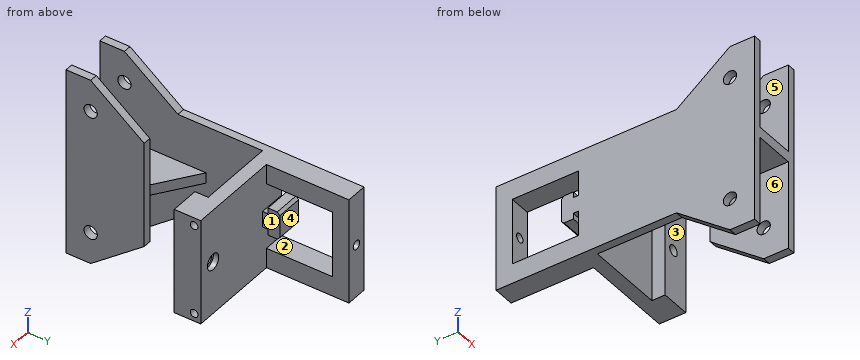
Autodesk Inventor part; units mm, degrees
ref_plane "YZ Plane" through (0, 0, 0) normal (1, 0, 0) x (0, 1, 0)
ref_plane "XZ Plane" through (0, 0, 0) normal (0, 1, 0) x (-1, 0, 0)
ref_plane "XY Plane" through (0, 0, 0) normal (0, 0, 1) x (1, 0, 0)
sketch "Szkic1" plane through (0, 0, 0) normal (1, 0, 0) x (0, 1, 0)
  line L0 (81.6216, 12.5) -> (106.6216, 12.5)
  line L1 (106.6216, 12.5) -> (106.6216, -12.5)
  line L2 (106.6216, -12.5) -> (81.6216, -12.5)
  line L3 (81.6216, -12.5) -> (81.6216, 12.5)
  line L4 (81.6216, 12.5) -> (106.6216, -12.5) construction
  line L5 (106.6216, 12.5) -> (81.6216, -12.5) construction
  line L6 (112.7335, 0) -> (112.7335, 20)
  line L7 (112.7335, 20) -> (44.7131, 20)
  line L8 (44.7131, 20) -> (24.5326, 35.4833)
  line L9 (24.5326, 35.4833) -> (15.2555, 35.4833)
  line L10 (15.2555, 35.4833) -> (15.2555, 0)
  line L11 (112.7335, 0) -> (112.7335, -20)
  line L12 (112.7335, -20) -> (44.7131, -20)
  line L13 (44.7131, -20) -> (24.5326, -35.4833)
  line L14 (24.5326, -35.4833) -> (15.2555, -35.4833)
  line L15 (15.2555, -35.4833) -> (15.2555, 0)
  point P0 (0, 0)
  point P1 (94.1216, 0)
  point P2 (24.5326, 19.6832)
  point P3 (24.5326, -19.6832)
  dimension "d0" = 25
  dimension "d1" = 25
  dimension "d2" = 82.089
  dimension "d3" = 20
extrude "Wyciągnięcie proste1" add sketch "Szkic1" along normal blind 3
sketch "Szkic2" plane through (3, 0, 0) normal (1, 0, 0) x (0, 0, -1)
  line L0 (-12.5, 106.6216) -> (12.5, 106.6216)
  line L1 (-35.4833, 24.5326) -> (-35.4833, 15.2555)
  line L2 (35.4833, 15.2555) -> (35.4833, 24.5326)
  point P0 (0, 0)
  point P1 (-23.4833, 24.5326)
  point P2 (23.4833, 24.5326)
  dimension "d6" = 82.089
  dimension "d7" = 82.089
  dimension "d8" = 12
  dimension "d9" = 12
hole "Otwór1" at (3, 24.5326, 23.4833) at (3, 24.5326, -23.4833) direction (-1, 0, 0) diameter 5 depth 3
sketch "Szkic3" plane through (3, 0, 0) normal (1, 0, 0) x (0, 0, -1)
  line L0 (-12.5, 106.6216) -> (12.5, 106.6216)
  line L1 (-12.5, 106.6216) -> (-20, 106.6216)
  line L2 (-20, 112.7335) -> (-20, 44.7131)
  line L3 (-12.5, 81.6216) -> (-12.5, 106.6216)
  line L4 (-20, 81.6216) -> (-12.5, 81.6216)
  line L5 (-12.5, 81.6216) -> (-12.5, 106.6216)
  line L6 (12.5, 106.6216) -> (12.5, 81.6216)
  line L7 (12.5, 106.6216) -> (12.5, 81.6216)
  line L8 (12.5, 81.6216) -> (20, 81.6216)
  line L9 (20, 81.6216) -> (20, 106.6216)
  line L10 (20, 106.6216) -> (12.5, 106.6216)
  line L11 (20, 44.7131) -> (20, 112.7335)
  point P0 (0, 0)
  point P1 (-20, 81.6216)
  dimension "d36" = 0
extrude "Wyciągnięcie proste2" add sketch "Szkic3" along normal blind 5
sketch "Szkic5" plane through (3, 0, 0) normal (1, 0, 0) x (0, 0, -1)
  line L0 (-35.4833, 15.2555) -> (35.4833, 15.2555)
  line L1 (0, 15.2555) -> (-2, 15.2555)
  line L2 (-2, 15.2555) -> (-2, 55.2555)
  line L3 (-2, 55.2555) -> (2, 55.2555)
  line L4 (2, 55.2555) -> (2, 15.2555)
  line L5 (0, 15.2555) -> (2, 15.2555)
  point P0 (0, 0)
  dimension "d26" = 2
  dimension "d27" = 40
  dimension "d28" = 4
extrude "Wyciągnięcie proste3" add sketch "Szkic5" along normal blind 15
sketch "Szkic6" plane through (18, 0, 0) normal (1, 0, 0) x (0, 0, -1)
  line L0 (-35.4833, 15.2555) -> (35.4833, 15.2555)
  line L1 (35.4833, 15.2555) -> (35.4833, 24.5326)
  line L2 (-35.4833, 15.2555) -> (35.4833, 15.2555)
  line L3 (35.4833, 15.2555) -> (35.4833, 24.5326)
  line L4 (35.4833, 24.5326) -> (20, 44.7131)
  line L5 (35.4833, 24.5326) -> (20, 44.7131)
  line L6 (-20, 44.7131) -> (-35.4833, 24.5326)
  line L7 (20, 44.7131) -> (-20, 44.7131)
  line L8 (-35.4833, 24.5326) -> (-35.4833, 15.2555)
  line L9 (-20, 44.7131) -> (-35.4833, 24.5326)
  line L10 (-35.4833, 24.5326) -> (-35.4833, 15.2555)
  circle A0 centre (-23.4833, 24.5326) radius 2.5
  circle A1 centre (23.4833, 24.5326) radius 2.5
  point P0 (0, 0)
extrude "Wyciągnięcie proste4" add sketch "Szkic6" along normal blind 3
chamfer "Faza1" distance 10.542 distance2 15 1 edges at (18, 55.2555, 0) measured on face at (18, 51.7413, 0.6667)
sketch "Szkic7" plane through (3, 0, 0) normal (1, 0, 0) x (0, 0, -1)
  line L0 (-20, 81.6216) -> (-12.5, 81.6216)
  line L1 (20, 44.7131) -> (20, 112.7335)
  line L2 (-20, 81.6216) -> (20, 81.6216)
  line L3 (20, 81.6216) -> (20, 76.6216)
  line L4 (20, 76.6216) -> (-20, 76.6216)
  line L5 (-20, 76.6216) -> (-20, 81.6216)
  point P0 (0, 0)
  dimension "d37" = 5
extrude "Wyciągnięcie proste5" add sketch "Szkic7" along normal blind 40
sketch "Szkic8" plane through (0, 81.6216, 12.5) normal (0, 1, 0) x (1, 0, 0)
  point P0 (0, 12.5)
  point P1 (36.4571, 12.5)
hole "Otwór3" at (36.4571, 81.6216, 0) direction (0, -1, 0) diameter 4 end through all
sketch "Szkic9" plane through (3, 0, 0) normal (1, 0, 0) x (0, 0, -1)
  line L0 (20, 112.7335) -> (-20, 112.7335)
  line L1 (20, 106.6216) -> (12.5, 106.6216)
  line L2 (-20, 112.7335) -> (20, 112.7335)
  line L3 (20, 112.7335) -> (20, 106.6216)
  line L4 (20, 106.6216) -> (-20, 106.6216)
  line L5 (-20, 106.6216) -> (-20, 112.7335)
  point P0 (0, 0)
extrude "Wyciągnięcie proste6" add sketch "Szkic9" along normal up to surface (5 mm away)
sketch "Szkic10" plane through (0, 0, 0) normal (-1, 0, 0) x (0, 0, 1)
  line L0 (-3.025, 81.6216) -> (-3.025, 83.6216)
  line L1 (-3.025, 83.6216) -> (-5.25, 83.6216)
  line L2 (-5.25, 83.6216) -> (-5.25, 87.1216)
  line L3 (0, 88.1216) -> (-4.25, 88.1216)
  line L4 (-4.25, 88.1216) -> (-5.25, 87.1216)
  line L5 (0, 88.1216) -> (4.25, 88.1216)
  line L6 (4.25, 88.1216) -> (5.25, 87.1216)
  line L7 (5.25, 83.6216) -> (5.25, 87.1216)
  line L8 (3.025, 83.6216) -> (5.25, 83.6216)
  line L9 (3.025, 81.6216) -> (3.025, 83.6216)
  line L10 (-12.5, 81.6216) -> (12.5, 81.6216)
  point P0 (0, 0)
  point P1 (0, 81.6216)
  point P2 (0, 81.6216)
  point P3 (-3.025, 82.6216)
  dimension "d49" = 2
  dimension "d50" = 2.225
  dimension "d51" = 3.5
  dimension "d52" = 4.25
  dimension "d53" = 0
  dimension "d54" = 3.025
extrude "Wyciągnięcie proste7" add sketch "Szkic10" against normal blind 10
sketch "Szkic11" plane through (0, 112.7335, 20) normal (0, 1, 0) x (1, 0, 0)
  point P0 (0, 20)
  point P1 (4, 20)
hole "Otwór4" at (4, 112.7335, 0) direction (0, -1, 0) diameter 3.4 depth 6.1119
sketch "Szkic13" plane through (3, 76.6216, -20) normal (0, -1, 0) x (1, 0, 0)
  line L0 (0, 0) -> (40, 0)
  line L1 (40, 40) -> (29, 40)
  line L2 (29, 40) -> (29, 0)
  line L3 (29, 0) -> (40, 0)
  line L4 (40, 0) -> (40, 40)
  point P0 (-3, 20)
  dimension "d65" = 11
extrude "Wyciągnięcie proste8" add sketch "Szkic13" along normal blind 5
sketch "Szkic14" plane through (0, 81.6216, 12.5) normal (0, 1, 0) x (1, 0, 0)
  circle A0 centre (36.4571, 12.5) radius 2
  circle A1 centre (36.4571, 12.5) radius 2
  point P0 (0, 12.5)
extrude "Wyciągnięcie proste9" cut sketch "Szkic14" against normal blind 10
sketch "Szkic15" plane through (0, 81.6216, 12.5) normal (0, 1, 0) x (1, 0, 0)
  circle A0 centre (36.4571, 12.5) radius 2
  circle A1 centre (36.4571, 12.5) radius 3
  point P0 (0, 12.5)
  dimension "d70" = 6
extrude "Wyciągnięcie proste10" cut sketch "Szkic15" against normal blind 2
sketch "Szkic16" plane through (43, 0, 0) normal (1, 0, 0) x (0, 0, -1)
  line L0 (20, 81.6216) -> (-20, 81.6216)
  line L1 (-20, 81.6216) -> (-20, 71.6216)
  line L2 (20, 81.6216) -> (20, 71.6216)
  point P0 (0, 0)
  point P1 (-17, 79.1216)
  point P2 (17, 79.1216)
  dimension "d73" = 2.5
  dimension "d74" = 3
  dimension "d75" = 2.5
  dimension "d76" = 3
hole "Otwór5" at (43, 79.1216, 17) at (43, 79.1216, -17) direction (-1, 0, 0) diameter 2.9 depth 14 tip angle 118
properties part number "równoważnia"
The model under review builds one solid part; all positions refer to its coordinate system, in mm. Face numbers are marked on the shaded views. A direction names the side the tool comes from. Coordinates: 2 decimals unless noted, no trailing zeros. Order: outer loops, then holes, each group sorted by start corner. A loop starts at its lowest first (then second) coordinate and runs counter-clockwise, first axis right, second up. Notation, with made-up numbers: (70, 75) -> (117, 75) arc R6 ccw to (117, 85) -> close; hole circle Ø7 at (2, 82.25). An arc over 180 degrees is marked (long way). Answer in a Markdown table with one row per item.
(1) Insertion check: pin 1 (1 mm diameter, centred on y = 38.5, z = -22.5, fed in from +X); pin 2 (3 mm diameter, centred on x = 5.5, y = 85, fed in from -Z); pin 3 (8 mm diameter, centred on x = 36.46, z = 0, fed in from -Y). Each pin has a flat end and moves straight along its axis. Give the tip position at first contact, or say it passes through.
Answers:
| item | result |
|---|---|
| pin 1 | x = 21 |
| pin 2 | z = -20 |
| pin 3 | y = 71.62 |
(2) Consider section B-B (y = 91). Write out the cut boundary in (x, z), plus the area to 3 significant figures.
Answers:
| item | result |
|---|---|
| outline | (0, -20) -> (8, -20) -> (8, -12.5) -> (0, -12.5) -> close; (0, 12.5) -> (8, 12.5) -> (8, 20) -> (0, 20) -> close |
| area | 120 mm² |
(3) Consider section C-C (x = 15). Write out the cut boundary in (y, z), plus the area to 3 significant figures.
Answers:
| item | result |
|---|---|
| outline | (15.26, -2) -> (46.82, -2) -> (46.82, 2) -> (15.26, 2) -> close; (76.62, -20) -> (81.62, -20) -> (81.62, 20) -> (76.62, 20) -> close |
| area | 326 mm² |
(4) The part is to be moulded in two halves that separate along Y. For the marked faces 1, 2 and 3, say which applies: +Y half, -Y half, draft (parallel to the pull), parting line (faces both ways), or undercut.
Answers:
| item | result |
|---|---|
| face 1 | draft |
| face 2 | undercut |
| face 3 | -Y half |
(5) Machinability: for the marked faces 4, 5 and 6, which of the approach directions +Z, -Z, +X, -X, +Y, -Y give a long, thin tool a straight path to every point of the face, cutting with its end or side? Answer none if there is none.
Answers:
| item | result |
|---|---|
| face 4 | +X, -X |
| face 5 | +Z, -Y |
| face 6 | -Z, -Y |
(6) Consider section A-A (z = 0). State how many separate pieces and enclosed holes the cut face has, plus the area to 3 significant figures.
Answers:
| item | result |
|---|---|
| separate pieces | 4 |
| enclosed holes | 0 |
| area | 1,110 mm² |
(7) Wall thickness on line 1 along X through (y, z) = (26.5, 29.5); line 2 along X through (y, z) = (110, 0); line 3 along X through (y, z) = (95, 17.5): over which ranges is each line inside the solid? List them lowest first.
Answers:
| item | result |
|---|---|
| line 1 | 0 to 3, 18 to 21 |
| line 2 | 0 to 2.3, 5.7 to 8 |
| line 3 | 0 to 8 |
(8) Consider section D-D (z = 11). Write out the cut boundary in (x, y), plus the area to 3 significant figures.
Answers:
| item | result |
|---|---|
| outline | (0, 15.26) -> (3, 15.26) -> (3, 76.62) -> (32, 76.62) -> (32, 71.62) -> (43, 71.62) -> (43, 81.62) -> (0, 81.62) -> close; (0, 106.62) -> (8, 106.62) -> (8, 112.73) -> (0, 112.73) -> close; (18, 15.26) -> (21, 15.26) -> (21, 44.71) -> (18, 44.71) -> close |
| area | 591 mm² |
